Design review of the part built by this model. Coordinates are the model's own, in mm. A direction names the side the tool comes from. Coordinates: 2 decimals unless noted, no trailing zeros. Loops run counter-clockwise (first coordinate to the right, second up) from the corner with the lowest first, then second, coordinate; pieces in that order, holes last. Notation, with made-up numbers: (58, 59) -> (117, 59) arc R31 ccw to (117, 94) -> close; hole circle Ø5 at (3.25, 61). An arc over 180 degrees is marked (long way). Answer in a Markdown table with one row per item.
```python
from build123d import *
from build123d import SkipClean  # not in build123d's __all__

# Parameters (mm, degrees)
F1_W          = 12.8
F1_H          = 25
F1_R          = 1.25
F2_DEPTH      = 8
F3_R          = 2.75
F4_DEPTH      = 8.001
F5_R          = 2
F6_DEPTH      = 2
F7_R          = 2.75
F8_DEPTH      = 1
F9_W          = 3
F9_H          = 6
F10_DEPTH     = 6
F11_W         = 4
F11_H         = 2
F12_DEPTH     = 3
F13_T1_DEPTH  = 2
F13_T3_DEPTH  = 2
F13_T8_DEPTH  = 4.5
F13_T13_DEPTH = 4.5
F13_T15_DEPTH = 8
F13_T17_DEPTH = 13
F14_R         = 4.5
F15_DEPTH     = 3


# Not quite as in the source:
# - a fillet or chamfer that OpenCascade refuses, or shapes differently, is made with other operations: its cross-section is extruded or revolved along the edge and cut away or added
# - after a boolean that leaves OpenCascade's solid faulty, fix() repairs it


with BuildPart() as f2:
    # F1 (on Front) → F2 (new body)
    with BuildSketch(Plane.XZ):
        with Locations((0, 9.25)):
            Rectangle(F1_W, F1_H)
        with Locations((-3.3, 1.75)):
            Circle(F1_R, mode=Mode.SUBTRACT)
        with Locations((3.2, 1.75)):
            Circle(F1_R, mode=Mode.SUBTRACT)
    extrude(amount=F2_DEPTH)

    # F3 (on face) → F4 (cut, through all)
    with BuildSketch(Plane(origin=(0, 0, 0), x_dir=(-1, 0, 0), z_dir=(0, 1, 0))):
        with Locations((0, 13.75)):
            Circle(F3_R)
    extrude(amount=-F4_DEPTH, mode=Mode.SUBTRACT)

    # F5 (on face) → F6 (cut)
    with BuildSketch(Plane.XZ.offset(8)):
        with Locations((-3.3, 1.75)):
            Circle(F5_R)
        with Locations((3.2, 1.75)):
            Circle(F5_R)
    extrude(amount=-F6_DEPTH, mode=Mode.SUBTRACT)

    # F7 (on face) → F8 (join)
    with BuildSketch(Plane.XZ.offset(8)):
        Polygon((-2.9, 5.75), (0, 5.75), (2.9, 5.75), (2.9, 21.75), (0, 21.75), (-2.9, 21.75), align=None)
        with Locations((0, 13.75)):
            Circle(F7_R, mode=Mode.SUBTRACT)
    with SkipClean():  # cleaning this boolean's faces spoils the solid; the shape is the same uncleaned
        extrude(amount=F8_DEPTH)

    # F9 (on face) → F10 (join)
    with BuildSketch(Plane.YZ.offset(6.4)):
        with Locations((-1.5, 9.75)):
            Rectangle(F9_W, F9_H)
    extrude(amount=F10_DEPTH)

    add(f2.part.fix(), mode=Mode.REPLACE)

    # F11 (on face) → F12 (cut, through all)
    with BuildSketch(Plane(origin=(0, 0, 0), x_dir=(-1, 0, 0), z_dir=(0, 1, 0))):
        with Locations((-8.4, 9.75)):
            Rectangle(F11_W, F11_H)
    extrude(amount=-F12_DEPTH, mode=Mode.SUBTRACT)

    add(f2.part.fix(), mode=Mode.REPLACE)

    # F13: fillet of radius 1 on 6 edges, made by hand

    # F13_s2 → F13_t1 (join)
    with BuildSketch(Plane.XY.offset(10.75)):
        with BuildLine():
            ThreePointArc((6.4, -4), (6.6928932188, -3.2928932188), (7.4, -3))
            Line((7.4, -3), (6.4, -3))
            Line((6.4, -3), (6.4, -4))
        make_face()
    extrude(amount=F13_T1_DEPTH)

    # F13_s4 → F13_t3 (join)
    with BuildSketch(Plane.XY.offset(6.75)):
        with BuildLine():
            ThreePointArc((6.4, -4), (6.6928932188, -3.2928932188), (7.4, -3))
            Line((7.4, -3), (6.4, -3))
            Line((6.4, -3), (6.4, -4))
        make_face()
    extrude(amount=F13_T3_DEPTH)


with BuildPart() as f13_tool6:
    # F13_s7 → F13_t8 (new body)
    with BuildSketch(Plane.XY.offset(12.75)):
        with BuildLine():
            ThreePointArc((6.4, -4), (6.6928932188, -3.2928932188), (7.4, -3))
            Line((7.4, -3), (6.4, -3))
            Line((6.4, -3), (6.4, -4))
        make_face()
    extrude(amount=-F13_T8_DEPTH)

    split(bisect_by=Plane.XY.offset(8.75), keep=Keep.BOTTOM)


with BuildPart() as f2_1:
    add(f2.part, clean=False)

    # F13_t5: union F13_tool6
    add(f13_tool6.part)


with BuildPart() as f13_tool11:
    # F13_s12 → F13_t13 (new body)
    with BuildSketch(Plane.XY.offset(11.25)):
        with BuildLine():
            ThreePointArc((6.4, -4), (6.6928932188, -3.2928932188), (7.4, -3))
            Line((7.4, -3), (6.4, -3))
            Line((6.4, -3), (6.4, -4))
        make_face()
    extrude(amount=-F13_T13_DEPTH)

    split(bisect_by=Plane.XY.offset(10.75), keep=Keep.TOP)


with BuildPart() as f2_2:
    add(f2_1.part, clean=False)

    # F13_t10: union F13_tool11
    add(f13_tool11.part)

    # F13_s16 → F13_t15 (cut)
    with BuildSketch(Plane.XZ.offset(-2.5)):
        with BuildLine():
            ThreePointArc((11.4, 6.75), (12.1071067812, 7.0428932188), (12.4, 7.75))
            Line((12.4, 7.75), (12.4, 6.75))
            Line((12.4, 6.75), (11.4, 6.75))
        make_face()
        with BuildLine():
            ThreePointArc((11.4, 12.75), (12.1071067812, 12.4571067812), (12.4, 11.75))
            Line((12.4, 11.75), (12.4, 12.75))
            Line((12.4, 12.75), (11.4, 12.75))
        make_face()
    extrude(amount=F13_T15_DEPTH, mode=Mode.SUBTRACT)

    # F13_s18 → F13_t17 (cut)
    with BuildSketch(Plane.XZ.offset(-2.5)):
        with BuildLine():
            ThreePointArc((5.4, 21.75), (6.1071067812, 21.4571067812), (6.4, 20.75))
            Line((6.4, 20.75), (6.4, 21.75))
            Line((6.4, 21.75), (5.4, 21.75))
        make_face()
        with BuildLine():
            ThreePointArc((-5.4, 21.75), (-6.1071067812, 21.4571067812), (-6.4, 20.75))
            Line((-6.4, 20.75), (-6.4, 21.75))
            Line((-6.4, 21.75), (-5.4, 21.75))
        make_face()
    extrude(amount=F13_T17_DEPTH, mode=Mode.SUBTRACT)

    # F14 (on face) → F15 (cut)
    with BuildSketch(Plane(origin=(0, 0, 0), x_dir=(-1, 0, 0), z_dir=(0, 1, 0))):
        with Locations((0, 13.75)):
            Circle(F14_R)
    extrude(amount=-F15_DEPTH, mode=Mode.SUBTRACT)


solid = f2_2.part
```
(1) Take a section at B-B on x = 8.25. Give the boundary of the cut face in (y, z).
Evaluation:
| item | result |
|---|---|
| outline | (-3, 6.75) -> (0, 6.75) -> (0, 8.75) -> (-3, 8.75) -> close; (-3, 10.75) -> (0, 10.75) -> (0, 12.75) -> (-3, 12.75) -> close |
(2) To check wall thickness, follow probe 1 along X at (y, z) = (-2, 1.75); probe 2 along Z at (x, y) = (0, -8.45); probe 3 along Z at (x, y) = (0, -7). State the ranges of each line that lie inside material, in increasing order.
Evaluation:
| item | result |
|---|---|
| probe 1 | x = -6.4 to -4.55, -2.05 to 1.95, 4.45 to 6.4 |
| probe 2 | z = 5.75 to 11, 16.5 to 21.75 |
| probe 3 | z = -3.25 to 11, 16.5 to 21.75 |
(3) Take a section at A-A on z = 1.75. Give the boundary of the cut face in (x, y).
Evaluation:
| item | result |
|---|---|
| outline | (-6.4, -8) -> (-5.3, -8) -> (-5.3, -6) -> (-4.55, -6) -> (-4.55, 0) -> (-6.4, 0) -> close; (-2.05, -6) -> (-1.3, -6) -> (-1.3, -8) -> (1.2, -8) -> (1.2, -6) -> (1.95, -6) -> (1.95, 0) -> (-2.05, 0) -> close; (4.45, -6) -> (5.2, -6) -> (5.2, -8) -> (6.4, -8) -> (6.4, 0) -> (4.45, 0) -> close |
(4) Draft analysis for pull direction X (two halves, no side actions). For faces 1 (the flat face through (8, -2, 10.75)), 2 (the flat face through (2.9, -8.5, 13.6)), 3 (the flat face through (-1, 0, 9)), state which applies: pulls with the +X half, pulls with the -X half, needs draft (parallel to the pull), parting line crosses it, or undercut.
Evaluation:
| item | result |
|---|---|
| face 1 | undercut |
| face 2 | pulls with the +X half |
| face 3 | needs draft |
(5) Take a section at C-C on y = -5.5. Give the boundary of the cut face in (x, z), and give its area (3 significant figures).
Evaluation:
| item | result |
|---|---|
| outline | (-6.4, -3.25) -> (6.4, -3.25) -> (6.4, 20.75) arc R1 ccw to (5.4, 21.75) -> (-5.4, 21.75) arc R1 ccw to (-6.4, 20.75) -> close; hole circle Ø2.5 at (-3.3, 1.75); hole circle Ø5.5 at (0, 13.75); hole circle Ø2.5 at (3.2, 1.75) |
| area | 286 mm² |
(6) For pin 1 (6.5 mm diameter, centred on x = 0, z = 13.75, fed in from +Y); pin 2 (2 mm diameter, centred on x = 8, y = -2.5, fed in from -Z); pin 3 (1.5 mm diameter, centred on x = 9, z = 8.5, fed in from -Y), all flat-tipped, find the tip position at first contact; note any pin that passes through.
Evaluation:
| item | result |
|---|---|
| pin 1 | stops at y = -3 |
| pin 2 | stops at z = 6.75 |
| pin 3 | stops at y = -3 |
(7) Tool access review of faces 4 (the flat face through (8, -2, 8.75)), 5 (the flat face through (0, -4, 21.75)), 6 (the flat face through (-2, -3, 16)), 7 (the flat face through (4, -6, 3)): name each direction out of +Z, -Z, +X, -X, +Y, -Y from which nothing blocks a thin tool from reaching the whole face with its end or side.
Evaluation:
| item | result |
|---|---|
| face 4 | +Y, -Y |
| face 5 | +Z, +X, -X, +Y, -Y |
| face 6 | +Y |
| face 7 | -Y |
(8) Take a section at D-D on z = 13.75. Give the boundary of the cut face in (x, y).
Evaluation:
| item | result |
|---|---|
| outline | (-6.4, -8) -> (-2.9, -8) -> (-2.9, -9) -> (-2.75, -9) -> (-2.75, -3) -> (-4.5, -3) -> (-4.5, 0) -> (-6.4, 0) -> close; (2.75, -9) -> (2.9, -9) -> (2.9, -8) -> (6.4, -8) -> (6.4, 0) -> (4.5, 0) -> (4.5, -3) -> (2.75, -3) -> close |
